```python
from build123d import *

# Parameters (mm, degrees)
F0_W     = 76.2
F0_H     = 38.1
F1_DEPTH = 6.35
F6_W     = 6.35
F6_H     = 38.1
F7_DEPTH = 25.4
F9_DEPTH = 3.175


with BuildPart() as f1:
    # F0 (on Top) → F1 (new body)
    with BuildSketch(Plane.XY):
        Rectangle(F0_W, F0_H)
    extrude(amount=-F1_DEPTH)

    # F2 (on face) → F3 (revolve)
    with BuildSketch(Plane.XY):
        with BuildLine():
            Line((-31.9676950246, 9.525), (-31.9676950246, 15.875))
            ThreePointArc((-31.9676950246, 15.875), (-35.1426950246, 12.7), (-31.9676950246, 9.525))
        make_face()
        with BuildLine():
            Line((-31.9676950246, -3.175), (-31.9676950246, 3.175))
            ThreePointArc((-31.9676950246, 3.175), (-35.1426950246, 0), (-31.9676950246, -3.175))
        make_face()
        with BuildLine():
            Line((-31.9676950246, -15.875), (-31.9676950246, -9.525))
            ThreePointArc((-31.9676950246, -9.525), (-35.1426950246, -12.7), (-31.9676950246, -15.875))
        make_face()
    revolve(axis=Axis((-31.9676950246, 0, 0), (0, 1, 0)))

    # F2 (on face) → F4 (revolve)
    with BuildSketch(Plane.XY):
        with BuildLine():
            Line((-19.2676950246, 9.525), (-19.2676950246, 15.875))
            ThreePointArc((-19.2676950246, 15.875), (-22.4426950246, 12.7), (-19.2676950246, 9.525))
        make_face()
        with BuildLine():
            Line((-19.2676950246, -3.175), (-19.2676950246, 3.175))
            ThreePointArc((-19.2676950246, 3.175), (-22.4426950246, 0), (-19.2676950246, -3.175))
        make_face()
        with BuildLine():
            Line((-19.2676950246, -15.875), (-19.2676950246, -9.525))
            ThreePointArc((-19.2676950246, -9.525), (-22.4426950246, -12.7), (-19.2676950246, -15.875))
        make_face()
    revolve(axis=Axis((-19.2676950246, 0, 0), (0, 1, 0)))

    # F2 (on face) → F5 (revolve)
    with BuildSketch(Plane.XY):
        with BuildLine():
            Line((-6.5676950246, 9.525), (-6.5676950246, 15.875))
            ThreePointArc((-6.5676950246, 15.875), (-9.7426950246, 12.7), (-6.5676950246, 9.525))
        make_face()
        with BuildLine():
            Line((-6.5676950246, -3.175), (-6.5676950246, 3.175))
            ThreePointArc((-6.5676950246, 3.175), (-9.7426950246, 0), (-6.5676950246, -3.175))
        make_face()
        with BuildLine():
            Line((-6.5676950246, -15.875), (-6.5676950246, -9.525))
            ThreePointArc((-6.5676950246, -9.525), (-9.7426950246, -12.7), (-6.5676950246, -15.875))
        make_face()
    revolve(axis=Axis((-6.5676950246, -12.7, 0), (0, 1, 0)))

    # F6 (on face) → F7 (join)
    with BuildSketch(Plane.XY):
        with Locations((34.925, 0)):
            Rectangle(F6_W, F6_H)
    extrude(amount=F7_DEPTH)

    # F8 (on Front) → F9 (join, symmetric)
    with BuildSketch(Plane.XZ):
        Polygon((31.75, 0), (31.75, 22.6986259222), (2.0545818843, 0), align=None)
    extrude(amount=F9_DEPTH, both=True)


solid = f1.part
```
Can you work these out from the model? Positions are in its coordinate system, mm. A direction names the side the tool comes from. Round coordinates to 2 decimals unless told otherwise and drop trailing zeros. Order: outer loops, then holes, each group sorted by start corner. A loop starts at its lowest first (then second) coordinate and runs counter-clockwise, first axis right, second up. Notation, with made-up numbers: (70, -37.75) -> (112, -37.75) arc R25 cw to (112, -12.75) -> close; hole circle Ø9 at (10.5, -6.75). An arc over 180 degrees is marked (long way). Return JSON: item names as keys, results as strings. Group by question number.
1. Will these pins go through, and if not, where does the flat tip stop? pin 1 (2 mm diameter, centred on x = 5, y = 9.5, fed in from +Z); pin 2 (1.5 mm diameter, centred on y = -15, z = 1, fed in from -X); pin 3 (10 mm diameter, centred on x = -7.5, y = -9, fed in from +Z) (3 decimals); pin 4 (12 mm diameter, centred on y = 1.5, z = 3.5, fed in from -X).
2. Which directions (+Z, -Z, +X, -X, +Y, -Y) give clear straight access to the entire face, cutting with the end or side of a thin tool? Please do faces 1 (the face through (35, 0, 25.4)), 2 (the face through (23, 3.175, 6)).
3. I need wall thicknesses on line 1 (Z direction, x = -17, y = -8.5); line 2 (X direction, y = -17, z = 2); line 3 (Y direction, x = 11, z = 1.5) (3 decimals). Which ranges of each line are inside material? Lowest first, please. Write a range as [from, to].
4. We'd pull the mould along X, two halves only. Please class faces 3 (the face through (38.1, 0, 9)), 4 (the face through (23, -3.175, 6)), 5 (the face through (-4, 5, 0)), 6 (the face through (-38.1, 0, -3)): released by +X, released by -X, zero draft, split by the parting line, or undercut.
5. If we section it at B-B, the plane x = 12: Write out the boundary of the cut face in (y, z) (3 decimals).
6. If we section it at A-A, the plane z = 2: Count the separate pieces of the cut face and the enclosed holes in it, then the cut area to 3 significant figures.
7. If we section it at C-C, the plane y = -11: Write out the boundary of the cut face in (x, z), then the cut area to 3 significant figures.
8. If we section it at D-D, the plane z = 5.5: Write out the boundary of the cut face in (x, y) (3 decimals), then the cut area to 3 significant figures.
Output values:
{
 "1": {"pin 1": "z = 0", "pin 2": "x = -34.61", "pin 3": "z = 3.175", "pin 4": "x = -38.1"},
 "2": {"face 1": "+Z, +X, -X, +Y, -Y", "face 2": "+Z, -X, +Y"},
 "3": {"line 1": "[-6.35, 0]", "line 2": "[31.75, 38.1]", "line 3": "[-3.175, 3.175]"},
 "4": {"face 3": "released by +X", "face 4": "zero draft", "face 5": "undercut", "face 6": "released by -X"},
 "5": {"outline": "(-19.05, -6.35) -> (19.05, -6.35) -> (19.05, 0) -> (3.175, 0) -> (3.175, 7.602) -> (-3.175, 7.602) -> (-3.175, 0) -> (-19.05, 0) -> close"},
 "6": {"separate pieces": "10", "enclosed holes": "0", "area": "586 mm²"},
 "7": {"outline": "(-38.1, -6.35) -> (38.1, -6.35) -> (38.1, 25.4) -> (31.75, 25.4) -> (31.75, 0) -> (-3.89, 0) arc R2.68 ccw to (-9.25, 0) -> (-16.59, 0) arc R2.68 ccw to (-21.95, 0) -> (-29.29, 0) arc R2.68 ccw to (-34.65, 0) -> (-38.1, 0) -> close", "area": "679 mm²"},
 "8": {"outline": "(9.25, -3.175) -> (31.75, -3.175) -> (31.75, -19.05) -> (38.1, -19.05) -> (38.1, 19.05) -> (31.75, 19.05) -> (31.75, 3.175) -> (9.25, 3.175) -> close", "area": "385 mm²"}
}
